from build123d import *

# Parameters (mm, degrees)
SKETCH090_R   = 2
SKETCH090_R_2 = 1.5
SKETCH090_W   = 10
SKETCH090_H   = 5
PAD_DEPTH     = 5


with BuildPart() as part:
    # Sketch090 → Pad (new body)
    with BuildSketch(Plane.XY):
        with BuildLine():
            Line((24.5, -35), (21.5, -35))
            ThreePointArc((18.5, -32), (19.37868, -34.12132), (21.5, -35))
            Line((18.5, -32), (18.5, -11.6))
            ThreePointArc((25.5, -4.6), (20.550253, -6.650253), (18.5, -11.6))
            Line((25.5, -4.6), (310.5, -4.6))
            ThreePointArc((316.5, -10.6), (314.742641, -6.357359), (310.5, -4.6))
            Line((316.5, -10.6), (316.5, -20))
            Line((316.5, -20), (333, -20))
            Line((333, -20), (333, -2.3))
            Line((333, -2.3), (327, -2.3))
            ThreePointArc((327, 3.7), (324, 0.7), (327, -2.3))
            Line((327, 3.7), (333, 3.7))
            Line((333, 3.7), (333, 6.7))
            Line((333, 6.7), (337, 6.7))
            Line((337, 6.7), (337, 16.5))
            ThreePointArc((337, 16.5), (329.091883, 35.591883), (310, 43.5))
            Line((310, 43.5), (251, 43.5))
            Line((251, 43.5), (251, 39.5))
            Line((251, 39.5), (236.5, 39.5))
            Line((236.5, 39.5), (236.5, 43.5))
            Line((236.5, 43.5), (192.25, 43.5))
            Line((192.25, 43.5), (192.25, 39.5))
            Line((192.25, 39.5), (177.75, 39.5))
            Line((177.75, 39.5), (177.75, 43.5))
            Line((177.75, 43.5), (133.5, 43.5))
            Line((133.5, 43.5), (133.5, 39.5))
            Line((133.5, 39.5), (119, 39.5))
            Line((119, 39.5), (119, 43.5))
            Line((119, 43.5), (80.5, 43.5))
            Line((80.5, 43.5), (80.5, 39.5))
            Line((80.5, 39.5), (76.5, 39.5))
            Line((76.5, 39.5), (76.5, 43.5))
            Line((76.5, 43.5), (-6.5, 43.5))
            Line((-6.5, 43.5), (-30, 20))
            Line((-30, 20), (-30, 7.325415))
            ThreePointArc((-33.363129, 3.962285), (-30.985038, 4.947323), (-30, 7.325415))
            ThreePointArc((-33.363129, 3.962285), (-37.322286, 0), (-33.363129, -3.962285))
            ThreePointArc((-30, -5.355339), (-31.543017, -4.324328), (-33.363129, -3.962285))
            Line((-30, -5.355339), (-14, -21.355339))
            Line((-14, -21.355339), (-14, -32))
            Line((-14, -32), (-6.5, -32))
            Line((-6.5, -32), (-6.5, -65))
            Line((-6.5, -65), (24.5, -65))
            Line((24.5, -65), (24.5, -35))
        make_face()
        with Locations((78.5, 27.751426)):
            Circle(SKETCH090_R, mode=Mode.SUBTRACT)
        with Locations((-3.05, -41.5)):
            Circle(SKETCH090_R_2, mode=Mode.SUBTRACT)
        with Locations((84.5, 12.5)):
            Circle(SKETCH090_R_2, mode=Mode.SUBTRACT)
        with Locations((22.05, -58.5)):
            Circle(SKETCH090_R_2, mode=Mode.SUBTRACT)
        with Locations((72.5, 20.1)):
            Circle(SKETCH090_R_2, mode=Mode.SUBTRACT)
        with Locations((-33.363129, 0)):
            Circle(SKETCH090_R_2, mode=Mode.SUBTRACT)
        with Locations((-10.5, -27.55)):
            Circle(SKETCH090_R_2, mode=Mode.SUBTRACT)
        with Locations((14, -27.55)):
            Circle(SKETCH090_R_2, mode=Mode.SUBTRACT)
        with Locations((-3.05, 37)):
            Circle(SKETCH090_R_2, mode=Mode.SUBTRACT)
        with Locations((22.05, 20)):
            Circle(SKETCH090_R_2, mode=Mode.SUBTRACT)
        Polygon((66.42768, 17), (66.42768, 18.193898), (61.42768, 18.193898), (61.42768, 17), (58.42768, 17), (58.42768, 8), (61.42768, 8), (61.42768, 6.806102), (66.42768, 6.806102), (66.42768, 8), (76, 8), (76, 17), align=None, mode=Mode.SUBTRACT)
        with BuildLine():
            ThreePointArc((21.92031, -1.500002), (23.42, -2e-06), (21.92031, 1.499998))
            Line((21.92031, 1.499998), (16.92031, 1.5))
            ThreePointArc((16.92031, 1.5), (15.42031, 0), (16.92031, -1.5))
            Line((16.92031, -1.5), (21.92031, -1.500002))
        make_face(mode=Mode.SUBTRACT)
        with BuildLine():
            Line((-21.92031, 1.5), (-26.92031, 1.5))
            ThreePointArc((-26.92031, 1.5), (-28.42031, 0), (-26.92031, -1.5))
            Line((-26.92031, -1.5), (-21.92031, -1.5))
            ThreePointArc((-21.92031, -1.5), (-20.42, 0), (-21.92031, 1.5))
        make_face(mode=Mode.SUBTRACT)
        with Locations((152, 12.5)):
            Rectangle(SKETCH090_W, SKETCH090_H, mode=Mode.SUBTRACT)
        with Locations((308, 12.5)):
            Rectangle(SKETCH090_W, SKETCH090_H, mode=Mode.SUBTRACT)
        with BuildLine():
            Line((-5, -8), (0, -8))
            ThreePointArc((0, -8), (8, 0), (0, 8))
            Line((0, 8), (-5, 8))
            ThreePointArc((-5, 8), (-13, 0), (-5, -8))
        make_face(mode=Mode.SUBTRACT)
        with Locations((22.5, 12.5)):
            Rectangle(SKETCH090_W, SKETCH090_H, mode=Mode.SUBTRACT)
    extrude(amount=PAD_DEPTH)


solid = part.part
The listing builds one solid part. Answer for the finished solid, in the listing's coordinates (mm). A direction names the side the tool comes from. Coordinates: 2 decimals unless noted, no trailing zeros. Write each loop counter-clockwise with the first axis right and the second up, starting at its lowest first coordinate (ties: lowest second). Pieces come first, ordered by that corner, then holes. Notation, with made-up numbers: M 15,-20.75 L 71,-20.75 A17 ccw 71,-0.75 Z; hole C 78,25.5 d8. An arc over 180 degrees is marked long. Put each result on its own line as item: value. Start each with the question number.
1. A cutting plane is placed at A-A on x = 94.5. Write down the section's boundary in (y, z), then the cut area to 4 significant figures.
2. Flat-ended cylindrical pins translate along their axes: P1, Ø2, axis at x = 240, z = 2, coming from the +Y side; P2, Ø1.5, axis at x = 60, z = 2, coming from the -Y side; P3, Ø1.5, axis at y = -16.5, z = 3.5, coming from the -X side. Find the tip coordinate at first contact, or state that the pin passes through.
3. Which of the six approach directions +Z, -Z, +X, -X, +Y, -Y give full straight-line access (tool end or side, diameter ignored) to faces 1 (the flat face through (-18, 32, 2)), 2 (the cylindrical face through (8, 0, 2)), 3 (the cylindrical face through (314.789, -6.404, 2.465))?
4. For a pull along X with two mould halves and no side action, classify faces 4 (the flat face through (147, 26, 0)), 5 (the cylindrical face through (20.6, -6.6, 2.5)), 6 (the cylindrical face through (329.3, 35.38, 2.46)) as pulls with the +X half, pulls with the -X half, needs draft (parallel to the pull), parting line crosses it, or undercut.
5. Consider line 1 (X direction, y = 10.5, z = 1.3); line 2 (Y direction, x = -3.05, z = 2.5); line 3 (Y direction, x = -1.5, z = 2.55). Determine where each line is inside the solid, lowest interval first. Write a range as from..to.
6. A cutting plane is placed at B-B on z = 1.2. Count the separate pieces of the cut face and the enclosed holes in it, then the cut area to 3 significant figures.
Resolved:
1. outline: M -4.6,0 L 43.5,0 L 43.5,5 L -4.6,5 Z
1. area: 240.5 mm2
2. P1: stops at y = 39.5
2. P2: stops at y = -4.6
2. P3: stops at x = -19.61
3. face 1: +Z, -Z, -X, +Y
3. face 2: +Z, -Z
3. face 3: +Z, -Z, -Y
4. face 4: needs draft
4. face 5: undercut
4. face 6: pulls with the +X half
5. line 1: x = -30..17.5, 27.5..58.43, 76..147, 157..303, 313..337
5. line 2: y = -65..-43, -40..-8, 8..35.5, 38.5..43.5
5. line 3: y = -65..-8, 8..43.5
6. separate pieces: 1
6. enclosed holes: 17
6. area: 18,600 mm2
